from build123d import *

# Parameters (mm, degrees)
SKETCH_1_W           = 15
SKETCH_1_H           = 4
EXTRUDE_1_DEPTH      = 85
SKETCH_17_W          = 15
SKETCH_17_H          = 12
SKETCH_17_H_2        = 3
EXTRUDE_2_DEPTH      = 10
EXTRUDE_2_DEPTH_BACK = 14
SKETCH_18_W          = 13
SKETCH_18_H          = 24
CUT_EXTRUDE_4_DEPTH  = 14
SKETCH_20_W          = 4.536667306
SKETCH_20_H          = 15
SKETCH_20_W_2        = 4.536667307
CUT_EXTRUDE_6_DEPTH  = 18
SKETCH_21_R          = 2
CUT_EXTRUDE_7_DEPTH  = 39
SKETCH_22_R          = 3.3
CUT_EXTRUDE_8_DEPTH  = 4
CUT_EXTRUDE_9_DEPTH  = 4


with BuildPart() as part:
    # 草图1 → 凸台-拉伸1 (new body)
    with BuildSketch(Plane(origin=(0, 0, 0), x_dir=(1, 0, 0), z_dir=(0, 1, 0))):
        with Locations((-12.365471303, -4.287695046)):
            Rectangle(SKETCH_1_W, SKETCH_1_H)
    extrude(amount=EXTRUDE_1_DEPTH)

    # 草图17 → 凸台-拉伸2 (add, two sides)
    with BuildSketch(Plane(origin=(0, 0, 2.287695046), x_dir=(-1, 0, 0), z_dir=(0, 0, -1))) as extrude_2_sk:
        with Locations((12.365471303, 79)):
            Rectangle(SKETCH_17_W, SKETCH_17_H)
        with Locations((12.365471303, 86.5)):
            Rectangle(SKETCH_17_W, SKETCH_17_H_2)
    extrude(amount=EXTRUDE_2_DEPTH)
    extrude(extrude_2_sk.sketch, amount=-EXTRUDE_2_DEPTH_BACK)

    # 草图18 → 切除-拉伸4 (cut)
    with BuildSketch(Plane(origin=(0, 88, 0), x_dir=(1, 0, 0), z_dir=(0, 1, 0))):
        with Locations((-12.365471303, -4.287695046)):
            Rectangle(SKETCH_18_W, SKETCH_18_H)
    extrude(amount=-CUT_EXTRUDE_4_DEPTH, mode=Mode.SUBTRACT)

    # 草图20 → 切除-拉伸6 (cut)
    with BuildSketch(Plane.ZY.offset(19.865471303)):
        with Locations((-5.443971301, 80.5)):
            Rectangle(SKETCH_20_W, SKETCH_20_H)
        with Locations((14.019361393, 80.5)):
            Rectangle(SKETCH_20_W_2, SKETCH_20_H)
    extrude(amount=-CUT_EXTRUDE_6_DEPTH, mode=Mode.SUBTRACT)

    # 草图21 → 切除-拉伸7 (cut)
    with BuildSketch(Plane.ZY.offset(19.865471303)):
        with Locations((4.287695046, 85.015112755)):
            Circle(SKETCH_21_R)
    extrude(amount=-CUT_EXTRUDE_7_DEPTH, mode=Mode.SUBTRACT)

    # 草图22 → 切除-拉伸8 (cut)
    with BuildSketch(Plane(origin=(0, 0, 2.287695046), x_dir=(-1, 0, 0), z_dir=(0, 0, -1))):
        with Locations((12.365471303, 5)):
            Circle(SKETCH_22_R)
    extrude(amount=-CUT_EXTRUDE_8_DEPTH, mode=Mode.SUBTRACT)

    # 草图23 → 切除-拉伸9 (cut)
    with BuildSketch(Plane.XY.offset(6.287695046)):
        Polygon((-13.537897134, 59.896284907), (-13.537897134, 69.113447), (-15.026236811, 69.113447), (-17.687002319, 64.504865953), (-15.026236811, 59.896284907), align=None)
        Polygon((-9.704705795, 59.896284907), (-7.043940288, 64.504865953), (-9.704705795, 69.113447), (-11.283232075, 69.113447), (-11.283232075, 59.896284907), align=None)
        Polygon((-13.537897134, 43.671503457), (-13.537897134, 53.576980938), (-17.240881786, 51.439061752), (-17.240881786, 45.809422642), align=None)
        Polygon((-7.49006082, 51.439061752), (-11.283232075, 53.629050197), (-11.283232075, 43.619434197), (-7.49006082, 45.809422642), align=None)
        Polygon((-13.537897134, 29.143330966), (-13.537897134, 38.360493059), (-15.026236811, 38.360493059), (-17.687002319, 33.751912013), (-15.026236811, 29.143330966), align=None)
        Polygon((-9.704705795, 38.360493059), (-11.283232075, 38.360493059), (-11.283232075, 29.143330966), (-9.704705795, 29.143330966), (-7.043940288, 33.751912013), align=None)
        Polygon((-13.537897134, 14.814321043), (-13.537897134, 23.721128572), (-16.808445012, 21.832876874), (-16.808445012, 16.70257274), align=None)
        Polygon((-7.922497595, 21.832876874), (-11.283232075, 23.773197831), (-11.283232075, 14.762251783), (-7.922497595, 16.70257274), align=None)
    extrude(amount=-CUT_EXTRUDE_9_DEPTH, mode=Mode.SUBTRACT)


solid = part.part
Here's how the part is built. I have some questions about the finished solid (model axes, mm). A direction names the side the tool comes from. Round coordinates to 2 decimals unless told otherwise and drop trailing zeros. Order: outer loops, then holes, each group sorted by start corner. A loop starts at its lowest first (then second) coordinate and runs counter-clockwise, first axis right, second up. Notation, with made-up numbers: (35.25, 48.5) -> (54.25, 48.5) arc R38 cw to (54.25, 87.5) -> close; hole circle Ø10 at (-1.75, -37). An arc over 180 degrees is marked (long way). Use CSV: the item, a comma, the result in double quotes.
1. Thinking about a two-plate mould opening in Y: for faces 4 (the face through (-5.865, 81, 4)), 5 (the face through (-9.626, 15.719, 4.316)), 6 (the face through (-12, 0, 4)), which applies, pulls with the +Y half, pulls with the -Y half, needs draft (parallel to the pull), parting line crosses it, or undercut?
Recorded:
face 4,"needs draft"
face 5,"undercut"
face 6,"pulls with the -Y half"
2. I want a section at A-A on y = 5. List the corners of the cut face in (x, z) for me.
Recorded:
outline,"(-19.87, 2.29) -> (-15.67, 2.29) -> (-15.67, 6.29) -> (-19.87, 6.29) -> close; (-9.07, 2.29) -> (-4.87, 2.29) -> (-4.87, 6.29) -> (-9.07, 6.29) -> close"
3. Which directions (+Z, -Z, +X, -X, +Y, -Y) give clear straight access to the entire face, cutting with the end or side of a thin tool? Please do faces 1 (the face through (-15.42, 44.76, 4.32)), 2 (the face through (-12, 74, 4)), 3 (the face through (-12, 73, 0)).
Recorded:
face 1,"+Z, -Z"
face 2,"+Z, -Z, +Y"
face 3,"-Z, +X, -X, -Y"
4. I need wall thicknesses on line 1 along X through (y, z) = (34, 5.5); line 2 along Y through (x, z) = (-11, 3); line 3 along Y through (x, z) = (-14.25, 3.5). Which ranges of each line are inside material? Lowest first, please.
Recorded:
line 1,"x = -19.87 to -17.54, -13.54 to -11.28, -7.19 to -4.87"
line 2,"y = 0 to 2, 8 to 14.93, 23.61 to 29.14, 38.36 to 43.78, 53.47 to 59.9, 69.11 to 74"
line 3,"y = 0 to 2.29, 7.71 to 15.23, 23.31 to 29.14, 38.36 to 44.08, 53.17 to 59.9, 69.11 to 74"
5. I want a section at C-C on x = -12.25. List the corners of the cut face in (y, z) for me, and give its area (3 significant figures).
Recorded:
outline,"(0, 2.29) -> (1.7, 2.29) -> (1.7, 6.29) -> (0, 6.29) -> close; (8.3, 2.29) -> (73, 2.29) -> (73, -3.18) -> (74, -3.18) -> (74, 11.75) -> (73, 11.75) -> (73, 6.29) -> (8.3, 6.29) -> close"
area,"281 mm2"
6. I want a section at D-D on y = 47. List the corners of the cut face in (x, z) for me.
Recorded:
outline,"(-19.87, 2.29) -> (-17.24, 2.29) -> (-17.24, 6.29) -> (-19.87, 6.29) -> close; (-13.54, 2.29) -> (-11.28, 2.29) -> (-11.28, 6.29) -> (-13.54, 6.29) -> close; (-7.49, 2.29) -> (-4.87, 2.29) -> (-4.87, 6.29) -> (-7.49, 6.29) -> close"
7. I want a section at B-B on z = 9. List the corners of the cut face in (x, y) for me.
Recorded:
outline,"(-19.87, 73) -> (-4.87, 73) -> (-4.87, 88) -> (-5.87, 88) -> (-5.87, 74) -> (-18.87, 74) -> (-18.87, 88) -> (-19.87, 88) -> close"
8. I'm going to push flat-ended pins straight in: P1, Ø0.5, axis at x = -10, z = 5, coming from the +Y side; P2, Ø4, axis at x = -10, y = 28, coming from the +Z side; P3, Ø1, axis at y = 37.5, z = 0, coming from the +X side; P4, Ø5, axis at x = -14.5, z = 9, coming from the -Y side. Where does each tip first touch, or does it pass through?
Recorded:
P1,"stops at y = 74"
P2,"stops at z = 6.29"
P3,"passes through"
P4,"stops at y = 73"
